from build123d import *

# Parameters (mm, degrees)
SKETCH_1_W                         = 63
SKETCH_1_H                         = 53
SM_BASE_FLANGE_1_DEPTH             = 3
SM_EDGE_FLANGE_1_STRIP_W           = 13.4732
SM_EDGE_FLANGE_1_STRIP_H           = 3
SM_EDGE_FLANGE_1_STRIP_CUT_DEPTH   = 53
SM_EDGE_FLANGE_1_STRIP_2_W         = 13.4732
SM_EDGE_FLANGE_1_STRIP_2_H         = 3
SM_EDGE_FLANGE_1_STRIP_CUT_2_DEPTH = 53
SM_EDGE_FLANGE_1_DEPTH             = 53
SM_EDGE_FLANGE_1_BEND_DEPTH        = 53
SKETCH_16_R                        = 1.5
SKETCH_16_R_2                      = 6.5
EXTRUDE_1_DEPTH                    = 3
EXTRUDE_START                      = -3
SKETCH_21_R                        = 2
SKETCH_21_R_2                      = 6.5
EXTRUDE_5_DEPTH                    = 3
EXTRUDE_6_DEPTH                    = 3
SKETCH_23_W                        = 61.5268
SKETCH_23_H                        = 20
EXTRUDE_7_DEPTH                    = 3
SKETCH_17_R                        = 1.5
SKETCH_17_R_2                      = 17
CUT_EXTRUDE_1_DEPTH                = 98.546142927
FILLET_2_R                         = 15
FILLET_3_R                         = 3
SKETCH_24_R                        = 1.5
CUT_EXTRUDE_2_DEPTH                = 98.546142927


# Sheet-metal steps are written as plain solids
with BuildPart() as part:
    # Sketch 1 → 基体-法兰1 (new body)
    with BuildSketch(Plane.XY):
        Rectangle(SKETCH_1_W, SKETCH_1_H)
    extrude(amount=-SM_BASE_FLANGE_1_DEPTH)

    # 边线-法兰1 strip (across the edge) → 边线-法兰1 strip cut (cut)
    with BuildSketch(Plane(origin=(-31.5, 26.5, 0), x_dir=(1, 0, 0), z_dir=(0, -1, 0))):
        with Locations((-6, -1.5)):
            Rectangle(SM_EDGE_FLANGE_1_STRIP_W, SM_EDGE_FLANGE_1_STRIP_H)
    extrude(amount=SM_EDGE_FLANGE_1_STRIP_CUT_DEPTH, mode=Mode.SUBTRACT)

    # 边线-法兰1 strip 2 (across the edge) → 边线-法兰1 strip cut 2 (cut)
    with BuildSketch(Plane(origin=(31.5, -26.5, 0), x_dir=(-1, 0, 0), z_dir=(0, 1, 0))):
        with Locations((-6, -1.5)):
            Rectangle(SM_EDGE_FLANGE_1_STRIP_2_W, SM_EDGE_FLANGE_1_STRIP_2_H)
    extrude(amount=SM_EDGE_FLANGE_1_STRIP_CUT_2_DEPTH, mode=Mode.SUBTRACT)

    # 边线-法兰1 section (across the edge) → 边线-法兰1 (add)
    with BuildSketch(Plane(origin=(-31.5, 26.5, 0), x_dir=(1, 0, 0), z_dir=(0, -1, 0))):
        with BuildLine():
            Line((-3, 0.7366), (-3, 5))
            Line((-3, 5), (0, 5))
            Line((0, 5), (0, 0.7366))
            ThreePointArc((0, 0.7366), (0.215745145, 0.215745145), (0.7366, 0))
            Line((0.7366, 0), (0.7366, -3))
            ThreePointArc((0.7366, -3), (-1.905575199, -1.905575199), (-3, 0.7366))
        make_face()
    extrude(amount=SM_EDGE_FLANGE_1_DEPTH)

    # 边线-法兰1 section 2 (across the edge) → 边线-法兰1 bend (add)
    with BuildSketch(Plane(origin=(31.5, -26.5, 0), x_dir=(-1, 0, 0), z_dir=(0, 1, 0))):
        with BuildLine():
            Line((-3, 0.7366), (-3, 5))
            Line((-3, 5), (0, 5))
            Line((0, 5), (0, 0.7366))
            ThreePointArc((0, 0.7366), (0.215745145, 0.215745145), (0.7366, 0))
            Line((0.7366, 0), (0.7366, -3))
            ThreePointArc((0.7366, -3), (-1.905575199, -1.905575199), (-3, 0.7366))
        make_face()
    extrude(amount=SM_EDGE_FLANGE_1_BEND_DEPTH)

    # 草图16 → 凸台-拉伸1 (add)
    with BuildSketch(Plane.ZY.offset(34.5)):
        with BuildLine():
            Line((26.141494742, 55.766183603), (0.7366, 26.5))
            Line((0.7366, 26.5), (5, 26.5))
            Line((5, 26.5), (5, -2.149105668))
            Line((5, -2.149105668), (29.00460009, 25.503952559))
            ThreePointArc((29.00460009, 25.503952559), (62.906640519, 43.977974267), (26.141494742, 55.766183603))
        make_face()
        with Locations((50, 55.856406461)):
            Circle(SKETCH_16_R, mode=Mode.SUBTRACT)
        with Locations((26, 42)):
            Circle(SKETCH_16_R, mode=Mode.SUBTRACT)
        with Locations((34, 28.143593539)):
            Circle(SKETCH_16_R, mode=Mode.SUBTRACT)
        with Locations((50, 28.143593539)):
            Circle(SKETCH_16_R, mode=Mode.SUBTRACT)
        with Locations((42, 42)):
            Circle(SKETCH_16_R_2, mode=Mode.SUBTRACT)
        with Locations((34, 55.856406461)):
            Circle(SKETCH_16_R, mode=Mode.SUBTRACT)
        with Locations((58, 42)):
            Circle(SKETCH_16_R, mode=Mode.SUBTRACT)
    extrude(amount=-EXTRUDE_1_DEPTH)

    # 草图21 → 凸台-拉伸5 (add)
    # profile 1 of 2: a face of its own
    with BuildSketch(Plane(origin=(34.5, 0, 0), x_dir=(0, 0, -1), z_dir=(1, 0, 0)).offset(EXTRUDE_START)):
        with BuildLine():
            ThreePointArc((-26.141494742, 55.766183603), (-60.431186758, 52.06436062), (-45.007392809, 21.216458711))
            ThreePointArc((-45.007392809, 21.216458711), (-36.565322242, 21.715417735), (-29.00460009, 25.503952559))
            Line((-29.00460009, 25.503952559), (-22.449274565, 17.952283389))
            Line((-22.449274565, 17.952283389), (-5, -2.149105668))
            Line((-5, -2.149105668), (-5, 26.5))
            Line((-5, 26.5), (-0.7366, 26.5))
            Line((-0.7366, 26.5), (-26.141494742, 55.766183603))
        make_face()
        with Locations((-48, 31.607695155)):
            Circle(SKETCH_21_R, mode=Mode.SUBTRACT)
        with Locations((-36, 31.607695155)):
            Circle(SKETCH_21_R, mode=Mode.SUBTRACT)
        with Locations((-54, 42)):
            Circle(SKETCH_21_R, mode=Mode.SUBTRACT)
        with Locations((-48, 52.392304845)):
            Circle(SKETCH_21_R, mode=Mode.SUBTRACT)
        with Locations(Location((-42, 42, 0), (0, 0, 180))):
            Circle(SKETCH_21_R_2, mode=Mode.SUBTRACT)
        with Locations((-36, 52.392304845)):
            Circle(SKETCH_21_R, mode=Mode.SUBTRACT)
        with Locations((-30, 42)):
            Circle(SKETCH_21_R, mode=Mode.SUBTRACT)
    # profile 2 of 2: a face of its own
    with BuildSketch(Plane(origin=(34.5, 0, 0), x_dir=(0, 0, -1), z_dir=(1, 0, 0)).offset(EXTRUDE_START)):
        with BuildLine():
            ThreePointArc((-29.00460009, 25.503952559), (-36.565322242, 21.715417735), (-45.007392809, 21.216458711))
            Line((-45.007392809, 21.216458711), (-22.449274565, 17.952283389))
            Line((-22.449274565, 17.952283389), (-29.00460009, 25.503952559))
        make_face()
    extrude(amount=EXTRUDE_5_DEPTH)

    # 草图22 → 凸台-拉伸6 (add)
    with BuildSketch(Plane.ZY.offset(34.5)):
        with BuildLine():
            Line((22.449274565, 17.952283389), (45.007392809, 21.216458711))
            ThreePointArc((45.007392809, 21.216458711), (36.565322242, 21.715417735), (29.00460009, 25.503952559))
            Line((29.00460009, 25.503952559), (22.449274565, 17.952283389))
        make_face()
    extrude(amount=-EXTRUDE_6_DEPTH)

    # 草图23 → 凸台-拉伸7 (add)
    with BuildSketch(Plane(origin=(0, 0, -3), x_dir=(-1, 0, 0), z_dir=(0, 0, -1))):
        with Locations((0, -36.5)):
            Rectangle(SKETCH_23_W, SKETCH_23_H)
    extrude(amount=-EXTRUDE_7_DEPTH)

    # 草图17 → 切除-拉伸1 (cut, through all)
    with BuildSketch(Plane(origin=(0, 0, -3), x_dir=(-1, 0, 0), z_dir=(0, 0, -1))):
        with Locations((0, 0.75)):
            Circle(SKETCH_17_R)
        with Locations((0, -20)):
            Circle(SKETCH_17_R_2)
        with Locations((14.67246571, -5.32753429)):
            Circle(SKETCH_17_R)
        with Locations((20.75, -20)):
            Circle(SKETCH_17_R)
        with Locations((14.67246571, -34.67246571)):
            Circle(SKETCH_17_R)
        with Locations((0, -40.75)):
            Circle(SKETCH_17_R)
        with Locations((-14.67246571, -34.67246571)):
            Circle(SKETCH_17_R)
        with Locations((-20.75, -20)):
            Circle(SKETCH_17_R)
        with Locations((-14.67246571, -5.32753429)):
            Circle(SKETCH_17_R)
    extrude(amount=-CUT_EXTRUDE_1_DEPTH, mode=Mode.SUBTRACT)

    # 圆角2
    fillet_2_edges = [part.edges().sort_by_distance(p)[0] for p in [
        (-30.7634, -46.5, -1.5),
        (30.7634, -46.5, -1.5),
    ]]
    fillet(fillet_2_edges, radius=FILLET_2_R)

    # 圆角3
    fillet_3_edges = [part.edges().sort_by_distance(p)[0] for p in [
        (-33, -26.5, 5),
        (33, -26.5, 5),
    ]]
    fillet(fillet_3_edges, radius=FILLET_3_R)

    # 草图24 → 切除-拉伸2 (cut, through all)
    with BuildSketch(Plane(origin=(0, 0, -3), x_dir=(-1, 0, 0), z_dir=(0, 0, -1))):
        with Locations((10, 21.5)):
            Circle(SKETCH_24_R)
        with Locations((-10, 21.5)):
            Circle(SKETCH_24_R)
        with BuildLine():
            Line((-10, 15.5), (10, 15.5))
            ThreePointArc((10, 15.5), (14, 11.5), (10, 7.5))
            Line((10, 7.5), (-10, 7.5))
            ThreePointArc((-10, 7.5), (-14, 11.5), (-10, 15.5))
        make_face()
    extrude(amount=-CUT_EXTRUDE_2_DEPTH, mode=Mode.SUBTRACT)


solid = part.part
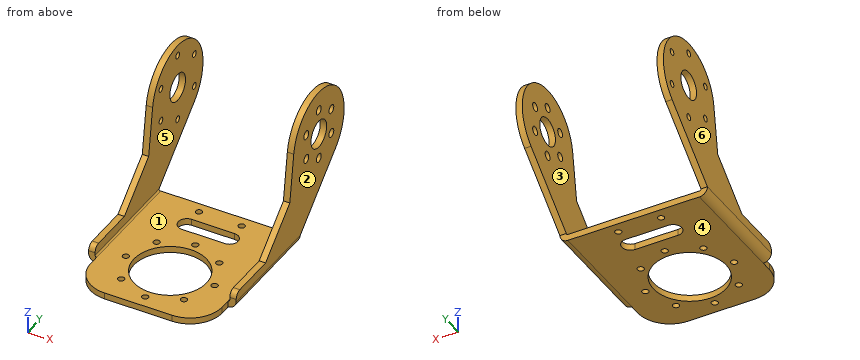
Build history of the part. All positions in model axes, mm. Face numbers are marked on the shaded views. A direction names the side the tool comes from. Round coordinates to 2 decimals unless told otherwise and drop trailing zeros. Write each loop counter-clockwise with the first axis right and the second up, starting at its lowest first coordinate (ties: lowest second). Pieces come first, ordered by that corner, then holes. Notation, with made-up numbers: (11.25, 77.5) -> (51.25, 77.5) arc R21 cw to (51.25, 82.5) -> close; hole circle Ø6 at (51, -13). An arc over 180 degrees is marked (long way). Write item = value, one per line.
(1) Band-saw the part on C-C (z = 54). Give the cut face in (x, y), then the cut area to 3 significant figures.
Answer:
outline = (-34.5, 24.77) -> (-31.5, 24.77) -> (-31.5, 59.23) -> (-34.5, 59.23) -> close; (31.5, 24.77) -> (34.5, 24.77) -> (34.5, 40) -> (31.5, 40) -> close; (31.5, 44) -> (34.5, 44) -> (34.5, 59.23) -> (31.5, 59.23) -> close
area = 195 mm2
(2) Probe L1, parallel to Y at x = 0, z = -0.7; L2, parallel to X at y = 27.5, z = 23; L3, parallel to Y at x = 10, z = -1. List the from-to ranges inside material, lowest first.
Answer:
L1 = -46.5 to -42.25, -39.25 to -37, -3 to -0.75, 2.25 to 7.5, 15.5 to 26.5
L2 = -34.5 to -31.5, 31.5 to 34.5
L3 = -46.5 to -33.75, -6.25 to 7.5, 15.5 to 20, 23 to 26.5
(3) Band-saw the part on D-D (x = -20.75). Give the cut face in (y, z).
Answer:
outline = (-45.65, -3) -> (-21.5, -3) -> (-21.5, 0) -> (-45.65, 0) -> close; (-18.5, -3) -> (26.5, -3) -> (26.5, 0) -> (-18.5, 0) -> close
(4) Band-saw the part on B-B (x = 0). Give the cut face in (y, z).
Answer:
outline = (-46.5, -3) -> (-42.25, -3) -> (-42.25, 0) -> (-46.5, 0) -> close; (-39.25, -3) -> (-37, -3) -> (-37, 0) -> (-39.25, 0) -> close; (-3, -3) -> (-0.75, -3) -> (-0.75, 0) -> (-3, 0) -> close; (2.25, -3) -> (7.5, -3) -> (7.5, 0) -> (2.25, 0) -> close; (15.5, -3) -> (26.5, -3) -> (26.5, 0) -> (15.5, 0) -> close
(5) Two-plate mould, pull along X, no slides. Class the marked faces 1, 2, 3 and 4: pulls with the +X half, pulls with the -X half, needs draft (parallel to the pull), parting line crosses it, or undercut.
Answer:
face_1 = undercut
face_2 = pulls with the +X half
face_3 = undercut
face_4 = needs draft
(6) Flat gauge pins, fed straight in: pin 1 (3.5 mm diameter, centred on y = -29.5, z = -1, fed in from +X); pin 2 (4 mm diameter, centred on x = -33, z = 0.5, fed in from -Y); pin 3 (0.9 mm diameter, centred on x = 3.5, z = -1.5, fed in from +Y). Where does each tip first touch, or does it go through?
Answer:
pin_1 = 30.76
pin_2 = -26.5
pin_3 = 26.5
(7) Band-saw the part on A-A (y = -20). Give the cut face in (x, z), then the cut area to 3 significant figures.
Answer:
outline = (-34.5, 0.74) arc R3.74 ccw to (-30.76, -3) -> (-22.25, -3) -> (-22.25, 0) -> (-30.76, 0) arc R0.74 cw to (-31.5, 0.74) -> (-31.5, 5) -> (-34.5, 5) -> close; (-19.25, -3) -> (-17, -3) -> (-17, 0) -> (-19.25, 0) -> close; (17, -3) -> (19.25, -3) -> (19.25, 0) -> (17, 0) -> close; (22.25, -3) -> (30.76, -3) arc R3.74 ccw to (34.5, 0.74) -> (34.5, 5) -> (31.5, 5) -> (31.5, 0.74) arc R0.74 cw to (30.76, 0) -> (22.25, 0) -> close
area = 111 mm2
(8) Tool access for the marked faces 5 and 6: list every direction of +Z, -Z, +X, -X, +Y, -Y with a clear straight run to the whole face (end or side of a thin tool).
Answer:
face_5 = +Z, +Y, -Y
face_6 = +Z, -Z, -X, +Y, -Y
